Design review of the part built by this model. Coordinates are the model's own, in mm. Face numbers are marked on the shaded views. A direction names the side the tool comes from. Coordinates: 2 decimals unless noted, no trailing zeros. Loops run counter-clockwise (first coordinate to the right, second up) from the corner with the lowest first, then second, coordinate; pieces in that order, holes last. Notation, with made-up numbers: (59, 30) -> (63, 30) arc R36 cw to (63, 69) -> close; hole circle Ø2 at (34.25, 49). An arc over 180 degrees is marked (long way). Use CSV: the item, a comma, the result in double quotes.
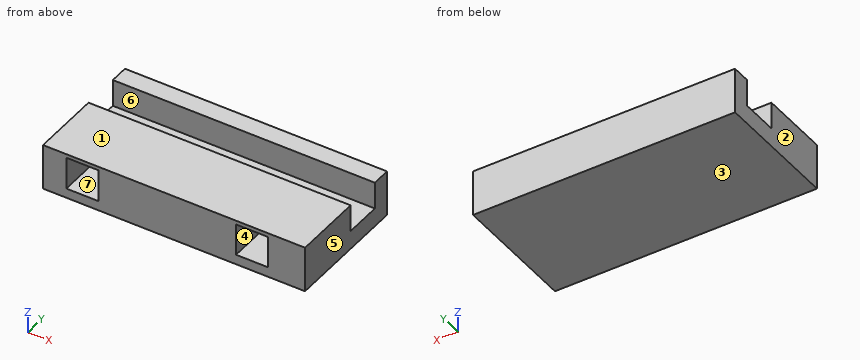
```python
from build123d import *

# Parameters (mm, degrees)
SKETCH1_W           = 27.99800038
SKETCH1_H           = 15
BOSS_EXTRUDE1_DEPTH = 4.9
SKETCH3_W           = 3.40799886
SKETCH3_H           = 3.410000155
SKETCH3_W_2         = 2.90799886
SKETCH3_H_2         = 2.910000155
SKETCH3_W_3         = 3.409995615
SKETCH3_H_3         = 3.468000248
SKETCH3_W_4         = 2.909995615
SKETCH3_H_4         = 2.968000248
CUT_EXTRUDE1_DEPTH  = 5.5
SKETCH4_W           = 2.9
SKETCH4_H           = 4
CUT_EXTRUDE2_DEPTH  = 30.5
SKETCH5_W           = 27.99800038
SKETCH5_H           = 4.9
CUT_EXTRUDE3_DEPTH  = 1.5


with BuildPart() as part:
    # Sketch1 → Boss-Extrude1 (new body)
    with BuildSketch(Plane.XY):
        with Locations((13.99900019, 7.5)):
            Rectangle(SKETCH1_W, SKETCH1_H)
    extrude(amount=BOSS_EXTRUDE1_DEPTH)

    # Sketch3 → Cut-Extrude1 (cut)
    # profile 1 of 4: a face of its own
    with BuildSketch(Plane.XZ):
        with Locations((22.329997268, 2.772999986)):
            Rectangle(SKETCH3_W, SKETCH3_H)
        with Locations((22.329997268, 2.772999986)):
            Rectangle(SKETCH3_W_2, SKETCH3_H_2, mode=Mode.SUBTRACT)
    # profile 2 of 4: a face of its own
    with BuildSketch(Plane.XZ):
        with Locations((22.329997268, 2.772999986)):
            Rectangle(SKETCH3_W_2, SKETCH3_H_2)
    # profile 3 of 4: a face of its own
    with BuildSketch(Plane.XZ):
        with Locations((4.200998691, 2.770000137)):
            Rectangle(SKETCH3_W_3, SKETCH3_H_3)
        with Locations((4.200998691, 2.770000137)):
            Rectangle(SKETCH3_W_4, SKETCH3_H_4, mode=Mode.SUBTRACT)
    # profile 4 of 4: a face of its own
    with BuildSketch(Plane.XZ):
        with Locations((4.200998691, 2.770000137)):
            Rectangle(SKETCH3_W_4, SKETCH3_H_4)
    extrude(amount=-CUT_EXTRUDE1_DEPTH, mode=Mode.SUBTRACT)

    # Sketch4 → Cut-Extrude2 (cut)
    with BuildSketch(Plane(origin=(27.99800038, 0, 0), x_dir=(0, 0, -1), z_dir=(1, 0, 0))):
        with Locations((-3.45, 9.5)):
            Rectangle(SKETCH4_W, SKETCH4_H)
    extrude(amount=-CUT_EXTRUDE2_DEPTH, mode=Mode.SUBTRACT)

    # Sketch5 → Cut-Extrude3 (cut)
    with BuildSketch(Plane(origin=(0, 15, 0), x_dir=(1, 0, 0), z_dir=(0, 1, 0))):
        with Locations((13.99900019, -2.45)):
            Rectangle(SKETCH5_W, SKETCH5_H)
    extrude(amount=-CUT_EXTRUDE3_DEPTH, mode=Mode.SUBTRACT)


solid = part.part
```
Item 1: Add section C-C (y = 2). Give the boundary of the cut face in (x, z), then the cut area to 3 significant figures.
Checked values:
outline,"(0, 0) -> (28, 0) -> (28, 4.9) -> (0, 4.9) -> close; hole (2.5, 1.04) -> (5.91, 1.04) -> (5.91, 4.5) -> (2.5, 4.5) -> close; hole (20.63, 1.07) -> (24.03, 1.07) -> (24.03, 4.48) -> (20.63, 4.48) -> close"
area,"114 mm^2"
Item 2: Draft analysis for pull direction Z (two halves, no side actions). For the marked faces 1, 2, 3 and 4, state which applies: pulls with the +Z half, pulls with the -Z half, needs draft (parallel to the pull), parting line crosses it, or undercut.
Checked values:
face 1,"pulls with the +Z half"
face 2,"needs draft"
face 3,"pulls with the -Z half"
face 4,"undercut"
Item 3: Clearance check with flat-ended pins moving along their axes: pin 1 (1 mm diameter, centred on x = 4, z = 3.5, fed in from -Y); pin 2 (1.2 mm diameter, centred on x = 8.5, y = 10, fed in from +Z). State where each tip first meets the part, or that it passes through.
Checked values:
pin 1,"y = 5.5"
pin 2,"z = 2"
Item 4: To check wall thickness, follow line 1 along X through (y, z) = (2.75, 3.55); line 2 along Y through (x, z) = (4.75, 3.85); line 3 along Y through (x, z) = (2.25, 2.95). State the ranges of each line that lie inside material, in increasing order.
Checked values:
line 1,"0 to 2.5, 5.91 to 20.63, 24.03 to 28"
line 2,"5.5 to 7.5, 11.5 to 13.5"
line 3,"0 to 7.5, 11.5 to 13.5"
Item 5: Add section D-D (x = 10). Give the boundary of the cut face in (y, z), then the cut area to 4 significant figures.
Checked values:
outline,"(0, 0) -> (13.5, 0) -> (13.5, 4.9) -> (11.5, 4.9) -> (11.5, 2) -> (7.5, 2) -> (7.5, 4.9) -> (0, 4.9) -> close"
area,"54.55 mm^2"
Item 6: Add section B-B (x = 21.25). Give the boundary of the cut face in (y, z), then the cut area to 3 significant figures.
Checked values:
outline,"(0, 0) -> (13.5, 0) -> (13.5, 4.9) -> (11.5, 4.9) -> (11.5, 2) -> (7.5, 2) -> (7.5, 4.9) -> (0, 4.9) -> (0, 4.48) -> (5.5, 4.48) -> (5.5, 1.07) -> (0, 1.07) -> close"
area,"35.8 mm^2"
Item 7: Machinability: for the marked faces 5, 6 and 7, which of the approach directions +Z, -Z, +X, -X, +Y, -Y give a long, thin tool a straight path to every point of the face, cutting with its end or side? Answer none if there is none.
Checked values:
face 5,"+Z, -Z, +X, +Y, -Y"
face 6,"+Z, +X, -X"
face 7,"-Y"
Item 8: Add section A-A (z = 2.65). Give the boundary of the cut face in (x, y).
Checked values:
outline,"(0, 0) -> (2.5, 0) -> (2.5, 5.5) -> (5.91, 5.5) -> (5.91, 0) -> (20.63, 0) -> (20.63, 5.5) -> (24.03, 5.5) -> (24.03, 0) -> (28, 0) -> (28, 7.5) -> (0, 7.5) -> close; (0, 11.5) -> (28, 11.5) -> (28, 13.5) -> (0, 13.5) -> close"
